CAD build for the part. Positions are in the model's coordinates, mm. A direction names the side the tool comes from. Give positions to 0.01 mm unless a question says otherwise; leave off trailing zeros. Order: outer loops, then holes, each group sorted by start corner. A loop starts at its lowest first (then second) coordinate and runs counter-clockwise, first axis right, second up.
from build123d import *

# Parameters (mm, degrees)
SKETCH1_R           = 30
BOSS_EXTRUDE1_DEPTH = 6
SKETCH2_R           = 9.75
BOSS_EXTRUDE2_DEPTH = 45
CUT_EXTRUDE1_DEPTH  = 67.340033162
SKETCH5_R           = 2.6
CUT_EXTRUDE3_DEPTH  = 30


with BuildPart() as part:
    # Sketch1 → Boss-Extrude1 (new body)
    with BuildSketch(Plane.XY):
        Circle(SKETCH1_R)
    extrude(amount=BOSS_EXTRUDE1_DEPTH)

    # Sketch2 → Boss-Extrude2 (add)
    with BuildSketch(Plane.XY.offset(6)):
        with Locations(Location((0, 0, 0), (0, 0, 180))):
            Circle(SKETCH2_R)
    extrude(amount=BOSS_EXTRUDE2_DEPTH)

    # Sketch3 → Cut-Extrude1 (cut, through all)
    with BuildSketch(Plane.XY.offset(51)):
        Polygon((0, 4.041451884), (-3.5, 2.020725942), (-3.5, -2.020725942), (0, -4.041451884), (3.5, -2.020725942), (3.5, 2.020725942), align=None)
    extrude(amount=-CUT_EXTRUDE1_DEPTH, mode=Mode.SUBTRACT)

    # Sketch5 → Cut-Extrude3 (cut)
    with BuildSketch(Plane(origin=(0, 0, 0), x_dir=(-1, 0, 0), z_dir=(0, 0, -1))):
        with Locations((0, 22.5)):
            Circle(SKETCH5_R)
        with Locations((19.485571585, 11.25)):
            Circle(SKETCH5_R)
        with Locations((19.485571585, -11.25)):
            Circle(SKETCH5_R)
        with Locations((0, -22.5)):
            Circle(SKETCH5_R)
        with Locations((-19.485571585, -11.25)):
            Circle(SKETCH5_R)
        with Locations((-19.485571585, 11.25)):
            Circle(SKETCH5_R)
    extrude(amount=-CUT_EXTRUDE3_DEPTH, mode=Mode.SUBTRACT)


solid = part.part
1. Saw through at A-A on z = 10.5. Give the cut face in (x, y).
2. Mould opens along Y. For faces 1 (the flat face through (-7.1, 7.1, 6)), 2 (the cylindrical face through (1.269, -9.667, 28.185)), 3 (the cylindrical face through (-21.887, -12.246, 2.958)) say: released by +Y, released by -Y, zero draft, split by the parting line, or undercut.
3. 3-axis set-ups, long thin cutter, end or side, ignore diameter. For faces 4 (the flat face through (-3.5, 0, 26)), 5 (the flat face through (-4, 0, 51)): which of +Z, -Z, +X, -X, +Y, -Y reach the whole face in a straight line?
4. Wall check: line 1 (Y direction, x = 0, z = 2.95); line 2 (X direction, y = 11, z = 3); line 3 (Z direction, x = 14.5, y = -10). Give the ranges that are in metal, low to high.
5. Pin check, flat tips, straight feed: P1, Ø3, axis at y = 0.5, z = 34.5, coming from the -X side; P2, Ø7, axis at x = 0, y = 22.5, coming from the +Z side; P3, Ø1.2, axis at y = -1, z = 24.5, coming from the +X side. Stop position of each tip, or through.
6. Saw through at D-D on y = 0. Give the cut face in (x, z).
7. Saw through at C-C on y = -11.25. Give the cut face in (x, z), plus the area to 3 significant figures.
8. Saw through at B-B on y = 24. Give the cut face in (x, z).
Reported:
1. outline: circle Ø19.5 at (0, 0); hole (-3.5, -2.02) - (0, -4.04) - (3.5, -2.02) - (3.5, 2.02) - (0, 4.04) - (-3.5, 2.02) - close
2. face 1: zero draft
2. face 2: split by the parting line
2. face 3: undercut
3. face 4: +Z, -Z
3. face 5: +Z, +X, -X, +Y, -Y
4. line 1: y = -30 to -25.1, -19.9 to -4.04, 4.04 to 19.9, 25.1 to 30
4. line 2: x = -27.91 to -22.07, -16.9 to 16.9, 22.07 to 27.91
4. line 3: z = 0 to 6
5. P1: stops at x = -9.75
5. P2: stops at z = 6
5. P3: stops at x = 9.74
6. outline: (-30, 0) - (-3.5, 0) - (-3.5, 51) - (-9.75, 51) - (-9.75, 6) - (-30, 6) - close; (3.5, 0) - (30, 0) - (30, 6) - (9.75, 6) - (9.75, 51) - (3.5, 51) - close
7. outline: (-27.81, 0) - (-22.09, 0) - (-22.09, 6) - (-27.81, 6) - close; (-16.89, 0) - (16.89, 0) - (16.89, 6) - (-16.89, 6) - close; (22.09, 0) - (27.81, 0) - (27.81, 6) - (22.09, 6) - close
7. area: 271 mm2
8. outline: (-18, 0) - (-2.12, 0) - (-2.12, 6) - (-18, 6) - close; (2.12, 0) - (18, 0) - (18, 6) - (2.12, 6) - close
